from build123d import *

# Parameters (mm, degrees)
SKETCH1_R           = 7
BOSS_EXTRUDE1_DEPTH = 25
SKETCH2_W           = 9
SKETCH2_H           = 30
BOSS_EXTRUDE2_DEPTH = 25
SKETCH3_R           = 3.6
CUT_EXTRUDE1_DEPTH  = 31.512292605


with BuildPart() as part:
    # Sketch1 → Boss-Extrude1 (new body)
    with BuildSketch(Plane(origin=(0, 0, 0), x_dir=(1, 0, 0), z_dir=(0, 1, 0))):
        with Locations(Location((0, 0, 0), (0, 0, 270))):
            Circle(SKETCH1_R)
    extrude(amount=BOSS_EXTRUDE1_DEPTH)

    # Sketch2 → Boss-Extrude2 (add)
    with BuildSketch(Plane(origin=(0, 25, 0), x_dir=(1, 0, 0), z_dir=(0, 1, 0))):
        with Locations((4.5, 0)):
            Rectangle(SKETCH2_W, SKETCH2_H)
    extrude(amount=-BOSS_EXTRUDE2_DEPTH)

    # Sketch3 → Cut-Extrude1 (cut, through all)
    with BuildSketch(Plane(origin=(0, 25, 0), x_dir=(1, 0, 0), z_dir=(0, 1, 0))):
        with Locations(Location((0, 0, 0), (0, 0, 270))):
            Circle(SKETCH3_R)
    extrude(amount=-CUT_EXTRUDE1_DEPTH, mode=Mode.SUBTRACT)


solid = part.part
The listing builds one solid part. Answer for the finished solid, in the listing's coordinates (mm). A direction names the side the tool comes from. Give positions to 0.01 mm unless a question says otherwise; leave off trailing zeros. Write each loop counter-clockwise with the first axis right and the second up, starting at its lowest first coordinate (ties: lowest second). Pieces come first, ordered by that corner, then holes. Notation, with made-up numbers: (34.5, -10) -> (53.5, -10) arc R23 ccw to (53.5, 26) -> close; hole circle Ø5 at (39.5, -7.5). An arc over 180 degrees is marked (long way). Use a Markdown table: item, result.
(1) Section C-C, the plane x = -2.75 is taken. Determine the outline of the cut face in (y, z).
Return value:
| item | result |
|---|---|
| outline | (0, -6.44) -> (25, -6.44) -> (25, -2.32) -> (0, -2.32) -> close; (0, 2.32) -> (25, 2.32) -> (25, 6.44) -> (0, 6.44) -> close |
(2) For faces 1 (the flat face through (0, 13, -11)), 2 (the flat face through (4, 25, 0)), determine the directions among +Z, -Z, +X, -X, +Y, -Y from which every point of the face is accessible in a straight line to the end or side of a thin tool.
Return value:
| item | result |
|---|---|
| face 1 | -Z, -X, +Y, -Y |
| face 2 | +Z, -Z, +X, -X, +Y |
(3) Find the intervals of material crossed by probe 1 along X at (y, z) = (14.5, 0); probe 2 along X at (y, z) = (12.5, 12.75); probe 3 along Z at (x, y) = (1.75, 5.75), in increasing order. Write a range as from..to.
Return value:
| item | result |
|---|---|
| probe 1 | -7..-3.6, 3.6..9 |
| probe 2 | 0..9 |
| probe 3 | -15..-3.15, 3.15..15 |
(4) Section D-D, the plane z = 6.5 is taken. Determine the outline of the cut face in (x, y).
Return value:
| item | result |
|---|---|
| outline | (-2.6, 0) -> (9, 0) -> (9, 25) -> (-2.6, 25) -> close |
(5) Determine the mould class of faces 3 (the cylindrical face through (-1.379, 12.675, 3.325)), 4 (the flat face through (0, 13, 11)), 5 (the flat face through (4, 13, 15)) for opening direction Z: released by +Z, released by -Z, zero draft, split by the parting line, or undercut.
Return value:
| item | result |
|---|---|
| face 3 | undercut |
| face 4 | zero draft |
| face 5 | released by +Z |
(6) Section A-A, the plane z = 0 is taken. Determine the outline of the cut face in (x, y), then the cut area to 3 significant figures.
Return value:
| item | result |
|---|---|
| outline | (-7, 0) -> (-3.6, 0) -> (-3.6, 25) -> (-7, 25) -> close; (3.6, 0) -> (9, 0) -> (9, 25) -> (3.6, 25) -> close |
| area | 220 mm2 |
(7) Flat-ended cylindrical pins translate along their axes: P1, Ø3, axis at y = 16, z = 4.5, coming from the -X side; P2, Ø8, axis at x = -3, y = 8.5, coming from the -Z side; P3, Ø2.5, axis at y = 10, z = -12, coming from the -X side. Find the tip coordinate at first contact, or state that the pin passes through.
Return value:
| item | result |
|---|---|
| P1 | x = -6.32 |
| P2 | z = -15 |
| P3 | x = 0 |
(8) Section B-B, the plane y = 6.75 is taken. Determine the outline of the cut face in (x, z).
Return value:
| item | result |
|---|---|
| outline | (0, -15) -> (9, -15) -> (9, 15) -> (0, 15) -> (0, 7) arc R7 ccw to (0, -7) -> close; hole circle Ø7.2 at (0, 0) |
